Could you check a few things on this model? Use its own coordinates, in mm. Face numbers are marked on the shaded views. A direction names the side the tool comes from. Round coordinates to 2 decimals unless told otherwise and drop trailing zeros. Write each loop counter-clockwise with the first axis right and the second up, starting at its lowest first coordinate (ties: lowest second). Pieces come first, ordered by that corner, then holes. Notation, with made-up numbers: (22.25, 19) -> (74.25, 19) arc R32 cw to (74.25, 58) -> close; hole circle Ø6 at (39, 46). An arc over 180 degrees is marked (long way). One line per question, with ' | ' between items. Start each with the question number.
1. Imagine slicing it at A-A, the plane z = 214.5. List the corners of the cut face in (x, y) for me, and give its area (3 significant figures).
2. For pin 1 Ø5 at (x, y) = (-319, 74) entering from -Z; pin 2 Ø6 at (x, y) = (-572.5, -218) entering from +Z; pin 3 Ø1.5 at (x, y) = (417, -223.5) entering from +Z, each with a flat end and sliding along its axis, tell me the tip position at first contact or that it passes through.
3. Imagine slicing it at B-B, the plane y = -160. List the corners of the cut face in (x, z) for me.
4. Imagine slicing it at C-C, the plane z = 78. List the corners of the cut face in (x, y) for me, and give its area (3 significant figures).
5. For the marked faces 4, 5 and 6, which set-ups out of +Z, -Z, +X, -X, +Y, -Y let a thin tool reach every point of the face, with its end or its side?
6. Thinking about a two-plate mould opening in Y: for the marked faces 1, 2 and 3, which applies, released by +Y, released by -Y, zero draft, split by the parting line, or undercut?
7. Imagine slicing it at D-D, the plane x = 331.5. List the corners of the cut face in (y, z) for me.
8. If I drill on line 1 along X through (y, z) = (-145, 425); line 2 along Y through (x, z) = (618, 868); line 3 along X through (y, z) = (-333, 922), over which ranges is the centre line in solid material (lowest first)? Write a range as [from, to].
from build123d import *

# Parameters (mm, degrees)
F0_W     = 1600
F0_H     = 1000
F1_DEPTH = 1000
F2_W     = 700
F2_H     = 800
F3_DEPTH = 900
F7_DEPTH = 600
F8_W     = 600.0000000002
F8_H     = 800
F9_DEPTH = 650


with BuildPart() as f1:
    # F0 (on Top) → F1 (new body)
    with BuildSketch(Plane.XY):
        Rectangle(F0_W, F0_H)
    extrude(amount=F1_DEPTH)

    # F2 (on face) → F3 (cut)
    with BuildSketch(Plane.XY.offset(1000)):
        with Locations((350, 0)):
            Rectangle(F2_W, F2_H)
    extrude(amount=-F3_DEPTH, mode=Mode.SUBTRACT)

    # F5 (on offset) → F7 (cut, through all)
    with BuildSketch(Plane(origin=(-700, 0, 0), x_dir=(0, -1, 0), z_dir=(-1, 0, 0))):
        Polygon((-400, 850), (400, 1000), (-400, 1000), align=None)
    extrude(amount=-F7_DEPTH, mode=Mode.SUBTRACT)

    # F8 (on face) → F9 (cut)
    with BuildSketch(Plane(origin=(0, 0, 0), x_dir=(1, 0, 0), z_dir=(0, 0, -1))):
        with Locations((-399.9999999999, 0)):
            Rectangle(F8_W, F8_H)
    extrude(amount=-F9_DEPTH, mode=Mode.SUBTRACT)


solid = f1.part
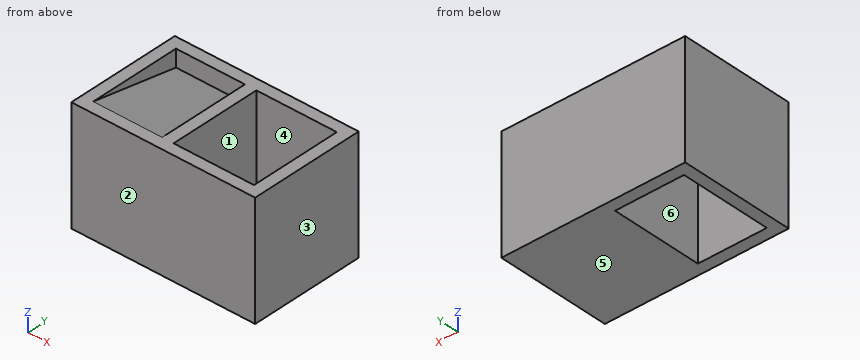
Geometry results:
1) outline: (-800, -500) -> (800, -500) -> (800, 500) -> (-800, 500) -> close; hole (-700, -400) -> (-100, -400) -> (-100, 400) -> (-700, 400) -> close; hole (0, -400) -> (700, -400) -> (700, 400) -> (0, 400) -> close | area: 560,000 mm2
2) pin 1: stops at z = 650 | pin 2: stops at z = 966.44 | pin 3: stops at z = 100
3) outline: (-800, 0) -> (-700, 0) -> (-700, 650) -> (-100, 650) -> (-100, 0) -> (800, 0) -> (800, 1000) -> (700, 1000) -> (700, 100) -> (0, 100) -> (0, 1000) -> (-100, 1000) -> (-100, 955) -> (-700, 955) -> (-700, 1000) -> (-800, 1000) -> close
4) outline: (-800, -500) -> (800, -500) -> (800, 500) -> (-800, 500) -> close; hole (-700, -400) -> (-100, -400) -> (-100, 400) -> (-700, 400) -> close | area: 1,120,000 mm2
5) face 4: +Z | face 5: -Z, +X, -X, +Y, -Y | face 6: -Z
6) face 1: undercut | face 2: released by -Y | face 3: zero draft
7) outline: (-500, 0) -> (500, 0) -> (500, 1000) -> (400, 1000) -> (400, 100) -> (-400, 100) -> (-400, 1000) -> (-500, 1000) -> close
8) line 1: x = [-800, -700], [-100, 0], [700, 800] | line 2: y = [-500, -400], [400, 500] | line 3: x = [-800, 0], [700, 800]
